The model under review builds one solid part; all positions refer to its coordinate system, in mm. Give positions to 0.01 mm unless a question says otherwise; leave off trailing zeros. Loops run counter-clockwise (first coordinate to the right, second up) from the corner with the lowest first, then second, coordinate; pieces in that order, holes last. Notation, with made-up numbers: M 8.25,35 L 57.25,35 A12 cw 57.25,58 Z; hole C -14,53 d1. An arc over 180 degrees is marked long. Return JSON: item names as keys, results as strings.
```python
from build123d import *

# Parameters (mm, degrees)
SKETCH_3_R      = 1.65
SKETCH_3_R_2    = 1.25
EXTRUDE_2_DEPTH = 3
FILLET_2_R      = 2


with BuildPart() as part:
    # 草图3 → 凸台-拉伸2 (new body)
    with BuildSketch(Plane.XY):
        with BuildLine():
            Line((9, 10), (0, 10))
            Line((0, 10), (0, 0))
            Line((0, 0), (75, 0))
            ThreePointArc((75, 0), (95.190046219, 36), (75, 72))
            Line((75, 72), (0, 72))
            Line((0, 72), (0, 62))
            Line((0, 62), (9, 62))
            Line((9, 62), (9, 10))
        make_face()
        with Locations((13.6, 8.6)):
            Circle(SKETCH_3_R, mode=Mode.SUBTRACT)
        with Locations((22.35, 8.6)):
            Circle(SKETCH_3_R, mode=Mode.SUBTRACT)
        with Locations((13.6, 18.35)):
            Circle(SKETCH_3_R, mode=Mode.SUBTRACT)
        with Locations((22.35, 18.35)):
            Circle(SKETCH_3_R, mode=Mode.SUBTRACT)
        with Locations((47.65, 8.6)):
            Circle(SKETCH_3_R, mode=Mode.SUBTRACT)
        with Locations((42.5, 17.813466521)):
            Circle(SKETCH_3_R_2, mode=Mode.SUBTRACT)
        with Locations((47.65, 21.35)):
            Circle(SKETCH_3_R, mode=Mode.SUBTRACT)
        with Locations((43, 26)):
            Circle(SKETCH_3_R, mode=Mode.SUBTRACT)
        with Locations((56.35, 8.6)):
            Circle(SKETCH_3_R, mode=Mode.SUBTRACT)
        with Locations((64, 13.65)):
            Circle(SKETCH_3_R, mode=Mode.SUBTRACT)
        with Locations((56.35, 21.35)):
            Circle(SKETCH_3_R, mode=Mode.SUBTRACT)
        with Locations((83, 17.813466521)):
            Circle(SKETCH_3_R, mode=Mode.SUBTRACT)
        with Locations((63, 26)):
            Circle(SKETCH_3_R, mode=Mode.SUBTRACT)
        with Locations((83, 26)):
            Circle(SKETCH_3_R, mode=Mode.SUBTRACT)
        with Locations((90.5, 31)):
            Circle(SKETCH_3_R, mode=Mode.SUBTRACT)
        with Locations((43, 46)):
            Circle(SKETCH_3_R, mode=Mode.SUBTRACT)
        with Locations((13.6, 53.65)):
            Circle(SKETCH_3_R, mode=Mode.SUBTRACT)
        with Locations((22.35, 53.65)):
            Circle(SKETCH_3_R, mode=Mode.SUBTRACT)
        with Locations((13.6, 63.4)):
            Circle(SKETCH_3_R, mode=Mode.SUBTRACT)
        with Locations((22.35, 63.4)):
            Circle(SKETCH_3_R, mode=Mode.SUBTRACT)
        with Locations((47.65, 50.65)):
            Circle(SKETCH_3_R, mode=Mode.SUBTRACT)
        with Locations((42.5, 54.186533479)):
            Circle(SKETCH_3_R_2, mode=Mode.SUBTRACT)
        with Locations((47.65, 63.4)):
            Circle(SKETCH_3_R, mode=Mode.SUBTRACT)
        with BuildLine():
            ThreePointArc((48.417424305, 26), (42, 36), (48.417424305, 46))
            ThreePointArc((48.417424305, 46), (64, 36), (48.417424305, 26))
        make_face(mode=Mode.SUBTRACT)
        with Locations((63, 46)):
            Circle(SKETCH_3_R, mode=Mode.SUBTRACT)
        with Locations((74, 36)):
            Circle(SKETCH_3_R_2, mode=Mode.SUBTRACT)
        with Locations((90.5, 41)):
            Circle(SKETCH_3_R, mode=Mode.SUBTRACT)
        with Locations((83, 46)):
            Circle(SKETCH_3_R, mode=Mode.SUBTRACT)
        with Locations((56.35, 50.65)):
            Circle(SKETCH_3_R, mode=Mode.SUBTRACT)
        with Locations((64, 56.35)):
            Circle(SKETCH_3_R, mode=Mode.SUBTRACT)
        with Locations((56.35, 63.4)):
            Circle(SKETCH_3_R, mode=Mode.SUBTRACT)
        with Locations((83, 56.35)):
            Circle(SKETCH_3_R, mode=Mode.SUBTRACT)
    extrude(amount=EXTRUDE_2_DEPTH)

    # 圆角2
    fillet_2_edges = [part.edges().sort_by_distance(p)[0] for p in [
        (0, 0, 1.5),
        (0, 10, 1.5),
        (9, 10, 1.5),
        (9, 62, 1.5),
        (0, 62, 1.5),
        (0, 72, 1.5),
    ]]
    fillet(fillet_2_edges, radius=FILLET_2_R)


solid = part.part
```
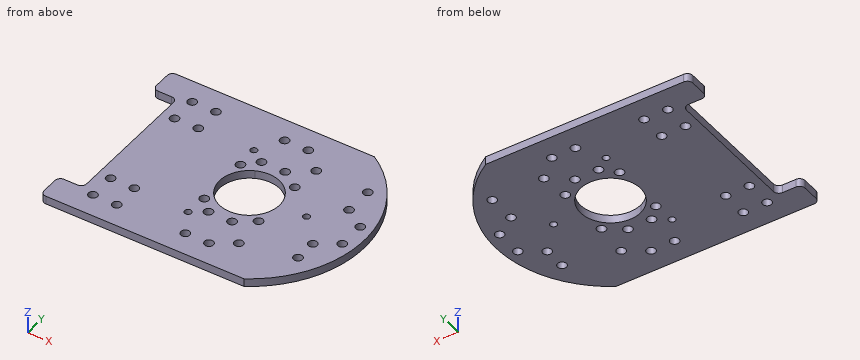
1) Consider section B-B on x = 83.5. Write out the cut boundary in (y, z), then the cut area to 3 significant figures.
From the geometry:
{"outline": "M 6.85,0 L 16.24,0 L 16.24,3 L 6.85,3 Z; M 19.39,0 L 24.43,0 L 24.43,3 L 19.39,3 Z; M 27.57,0 L 44.43,0 L 44.43,3 L 27.57,3 Z; M 47.57,0 L 54.78,0 L 54.78,3 L 47.57,3 Z; M 57.92,0 L 65.15,0 L 65.15,3 L 57.92,3 Z", "area": "137 mm²"}
2) Insertion check: pin 1 (1.5 mm diameter, centred on y = 50.5, z = 0.5, fed in from -X). The pin has a flat end and moves straight along its axis. Give the tip position at first contact, or say it passes through.
From the geometry:
{"pin 1": "x = 9"}
3) Consider section A-A on x = 53. Write out the cut boundary in (y, z).
From the geometry:
{"outline": "M 0,0 L 25,0 L 25,3 L 0,3 Z; M 47,0 L 72,0 L 72,3 L 47,3 Z"}
4) Consider section D-D on x = 23. Write out the cut boundary in (y, z).
From the geometry:
{"outline": "M 0,0 L 7.08,0 L 7.08,3 L 0,3 Z; M 10.12,0 L 16.83,0 L 16.83,3 L 10.12,3 Z; M 19.87,0 L 52.13,0 L 52.13,3 L 19.87,3 Z; M 55.17,0 L 61.88,0 L 61.88,3 L 55.17,3 Z; M 64.92,0 L 72,0 L 72,3 L 64.92,3 Z"}
5) Consider section C-C on z = 0.65. Count the separate pieces of the cut face and the enclosed holes in it, then the cut area to 3 significant figures.
From the geometry:
{"separate pieces": "1", "enclosed holes": "32", "area": "5,320 mm²"}
6) Wall thickness on L1, parallel to Y at x = 22.35, z = 1.65; L2, parallel to Y at x = 84, z = 0.5; L3, parallel to X at y = 51, z = 2.25: over which ranges is each line inside the solid? List them lowest first. Write a range as from..to.
From the geometry:
{"L1": "0..6.95, 10.25..16.7, 20..52, 55.3..61.75, 65.05..72", "L2": "7.38..16.5, 19.13..24.69, 27.31..44.69, 47.31..55.04, 57.66..64.62", "L3": "9..46.04, 49.26..54.74, 57.96..92.43"}
